Here's the drawing with two shaded views (mm, measured from the low corner). I have some questions. Give positions to 0.01 mm unless a question says otherwise; leave off trailing zeros. Write each loop counter-clockwise with the first axis right and the second up, starting at its lowest first coordinate (ties: lowest second). Pieces come first, ordered by that corner, then holes.
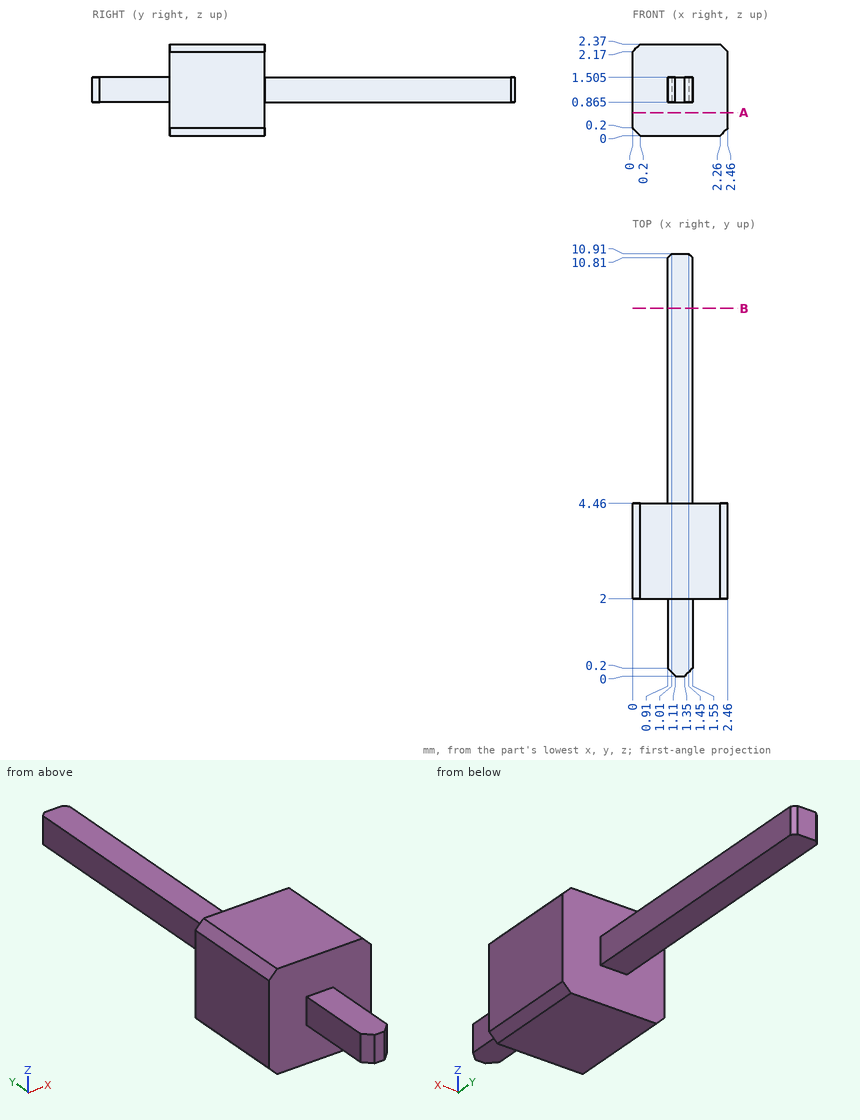
(1) Will these pins go through, and if not, where does the flat tip stop? P1, Ø0.7, axis at x = 1, y = 8.5, coming from the -Z side (3 decimals); P2, Ø0.5, axis at y = 1, z = 1, coming from the -X side; P3, Ø0.7, axis at x = 1, y = 1, coming from the +Z side (3 decimals).
Returned:
P1: stops at z = 0.865
P2: stops at x = 0.91
P3: stops at z = 1.505
(2) Imagine slicing it at B-B, the plane y = 9.5. Write out the boundary of the cut face in (x, z) (3 decimals), plus the area to 3 significant figures.
Returned:
outline: (0.91, 0.865) - (1.55, 0.865) - (1.55, 1.505) - (0.91, 1.505) - close
area: 0.410 mm2
(3) If I drill on L1, parallel to X at y = 9, z = 1; L2, parallel to Y at x = 0.75, z = 1.1; L3, parallel to Z at x = 0.95, y = 0.75 (3 decimals), over which ranges is the centre line in solid material (lowest first)?
Returned:
L1: x = 0.91 to 1.55
L2: y = 2 to 4.46
L3: z = 0.865 to 1.505
(4) Imagine slicing it at A-A, the plane z = 0.6. Write out the boundary of the cut face in (x, y).
Returned:
outline: (0, 2) - (2.46, 2) - (2.46, 4.46) - (0, 4.46) - close
